The model under review builds one solid part; all positions refer to its coordinate system, in mm. Face numbers are marked on the shaded views. A direction names the side the tool comes from. Coordinates: 2 decimals unless noted, no trailing zeros. Order: outer loops, then holes, each group sorted by start corner. A loop starts at its lowest first (then second) coordinate and runs counter-clockwise, first axis right, second up. Notation, with made-up numbers: (86, 17) -> (130, 17) arc R11 cw to (130, 31) -> close; hole circle Ø11 at (32.5, 51). An arc over 180 degrees is marked (long way). Use CSV: the item, a comma, the result in double quotes. Start each with the question number.
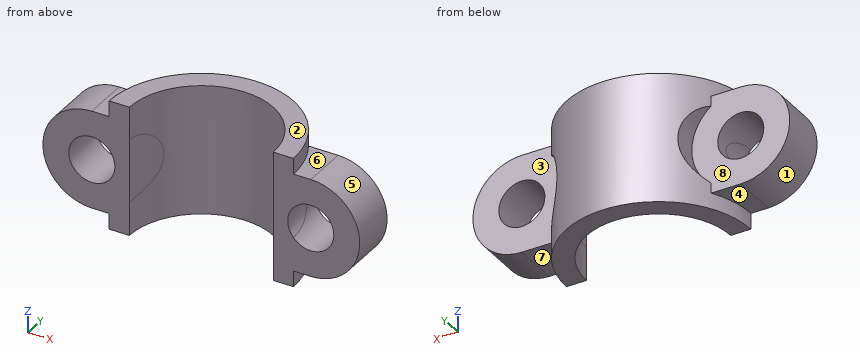
```python
from build123d import *

# Parameters (mm, degrees)
SKETCH_4_R          = 8.5
SKETCH_4_R_2        = 4
EXTRUDE_1_DEPTH     = 8
EXTRUDE_1_2_DEPTH   = 8
SKETCH_5_R          = 12.5
CUT_EXTRUDE_1_DEPTH = 10
EXTRUDE_3_DEPTH     = 11.25
SKETCH_7_R          = 8.5
CUT_EXTRUDE_2_DEPTH = 31.770318642
EXTRUDE_START       = -8
EXTRUDE_4_DEPTH     = 8
SKETCH_9_R          = 4
CUT_EXTRUDE_3_DEPTH = 31.770318642


with BuildPart() as part:
    # Sketch 4 → Extrude 1 (new body)
    with BuildSketch(Plane(origin=(0, 0, 0), x_dir=(1, 0, 0), z_dir=(0, 1, 0))):
        with Locations(Location((-19, 0, 0), (0, 0, 270))):
            Circle(SKETCH_4_R)
        with Locations(Location((-19, 0, 0), (0, 0, 270))):
            Circle(SKETCH_4_R_2, mode=Mode.SUBTRACT)
    extrude(amount=EXTRUDE_1_DEPTH)


with BuildPart() as body_2:
    # Sketch 4 → Extrude 1 2 (new body)
    with BuildSketch(Plane(origin=(0, 0, 0), x_dir=(1, 0, 0), z_dir=(0, 1, 0))):
        with Locations(Location((19, 0, 0), (0, 0, 90))):
            Circle(SKETCH_4_R)
        with Locations(Location((19, 0, 0), (0, 0, 90))):
            Circle(SKETCH_4_R_2, mode=Mode.SUBTRACT)
    extrude(amount=EXTRUDE_1_2_DEPTH)


with BuildPart() as cut_extrude_1_tool:
    # Sketch 5 → Cut-Extrude 1 (new, symmetric)
    with BuildSketch(Plane.XY):
        Circle(SKETCH_5_R)
    extrude(amount=CUT_EXTRUDE_1_DEPTH, both=True)


with BuildPart() as part_1:
    add(part.part)

    # Cut-Extrude 1: cut by cut_extrude_1_tool
    add(cut_extrude_1_tool.part, mode=Mode.SUBTRACT)



with BuildPart() as body_2_1:
    add(body_2.part)

    # Cut-Extrude 1: cut by cut_extrude_1_tool
    add(cut_extrude_1_tool.part, mode=Mode.SUBTRACT)


with BuildPart() as part_2:
    add(part_1.part)

    add(body_2_1.part)  # Extrude 3 merges body 2
    # Sketch 6 → Extrude 3 (add, symmetric)
    with BuildSketch(Plane.XY):
        with BuildLine():
            Line((-16, 0), (-12.5, 0))
            ThreePointArc((-12.5, 0), (0, 12.5), (12.5, 0))
            Line((12.5, 0), (16, 0))
            ThreePointArc((16, 0), (0, 16), (-16, 0))
        make_face()
    extrude(amount=EXTRUDE_3_DEPTH, both=True)

    # Sketch 7 → Cut-Extrude 2 (cut, through all)
    with BuildSketch(Plane(origin=(0, 8, 0), x_dir=(1, 0, 0), z_dir=(0, 1, 0))):
        with Locations((-19, 0)):
            Circle(SKETCH_7_R)
    cut_extrude_2 = extrude(amount=CUT_EXTRUDE_2_DEPTH, mode=Mode.SUBTRACT)

    # Sketch 8 → Extrude 4 (add)
    with BuildSketch(Plane(origin=(0, 8, 0), x_dir=(1, 0, 0), z_dir=(0, 1, 0)).offset(EXTRUDE_START)):
        with BuildLine():
            Line((-19, -8.5), (-19, -4))
            ThreePointArc((-19, -4), (-15, 0), (-19, 4))
            Line((-19, 4), (-19, 8.5))
            Line((-19, 8.5), (-13.461758669, 8.5))
            Line((-13.461758669, 8.5), (-13.461758669, -8.5))
            Line((-13.461758669, -8.5), (-19, -8.5))
        make_face()
    extrude_4 = extrude(amount=EXTRUDE_4_DEPTH)

    # Sketch 9 → Cut-Extrude 3 (cut, through all)
    with BuildSketch(Plane(origin=(0, 8, 0), x_dir=(1, 0, 0), z_dir=(0, 1, 0))):
        with Locations(Location((-19, 0, 0), (0, 0, 270))):
            Circle(SKETCH_9_R)
    cut_extrude_3 = extrude(amount=-CUT_EXTRUDE_3_DEPTH, mode=Mode.SUBTRACT)

    # Mirror 1: Cut-Extrude 2, Extrude 4, Cut-Extrude 3 across plane
    add(cut_extrude_2.mirror(Plane(origin=(0, 0, 0), x_dir=(0, 0, 1), z_dir=(1, 0, 0))), mode=Mode.SUBTRACT)
    add(extrude_4.mirror(Plane(origin=(0, 0, 0), x_dir=(0, 0, 1), z_dir=(1, 0, 0))))
    add(cut_extrude_3.mirror(Plane(origin=(0, 0, 0), x_dir=(0, 0, 1), z_dir=(1, 0, 0))), mode=Mode.SUBTRACT)


solid = part_2.part
```
Q1. Add section A-A, the plane z = 0. State the section outline as (x, y) points.
Q2. Add section C-C, the plane x = 0. State the section outline as (y, z) points, then the cut area to 4 significant figures.
Q3. Clearance check with flat-ended pins moving along their axes: pin 1 Ø2.5 at (x, y) = (16.5, 3.5) entering from +Z; pin 2 Ø5 at (x, z) = (20.5, 4) entering from +Y; pin 3 Ø1.5 at (x, y) = (-16.5, 5) entering from -Z; pin 4 Ø6 at (x, z) = (-5, 0) entering from +Y. State where each tip first meets the part, or that it passes through.
Q4. To check wall thickness, follow probe 1 along Z at (x, y) = (-19, 2.5); probe 2 along X at (y, z) = (2.75, 0.75); probe 3 along X at (y, z) = (5.25, 0). State the ranges of each line that lie inside material, in increasing order.
Q5. For the marked faces 4, 5, 6, 7 and 8, list the 3-axis set-ups (+Z, -Z, +X, -X, +Y, -Y) from which the entire face can be reached by the end or side of a thin tool; tool diameter is ignored.
Q6. Add section D-D, the plane y = 10.75. State the section outline as (x, z) points, then the cut area to 3 significant figures.
Q7. Draft analysis for pull direction Z (two halves, no side actions). For the marked faces 1, 2 and 3, state which applies: +Z half, -Z half, draft (parallel to the pull), parting line (faces both ways), or undercut.
Q8. Add section B-B, the plane y = 3. State the section outline as (x, z) points.
Answer block:
1,outline,"(-27.5, 0) -> (-23, 0) -> (-23, 8) -> (-27.5, 8) -> close; (-15, 0) -> (-12.5, 0) arc R12.5 cw to (12.5, 0) -> (15, 0) -> (15, 8) -> (10.5, 8) -> (10.5, 12.07) arc R16 ccw to (-10.5, 12.07) -> (-10.5, 8) -> (-15, 8) -> close; (23, 0) -> (27.5, 0) -> (27.5, 8) -> (23, 8) -> close"
2,outline,"(12.5, -11.25) -> (16, -11.25) -> (16, 11.25) -> (12.5, 11.25) -> close"
2,area,"78.75 mm²"
3,pin 1,"stops at z = 11.25"
3,pin 2,"stops at y = 8"
3,pin 3,"stops at z = -8.5"
3,pin 4,"stops at y = 15.87"
4,probe 1,"z = -8.5 to -4, 4 to 8.5"
4,probe 2,"x = -27.47 to -22.93, -15.07 to -12.19, 12.19 to 15.07, 22.93 to 27.47"
4,probe 3,"x = -27.5 to -23, -15 to -11.34, 11.34 to 15, 23 to 27.5"
5,face 4,"-Z, -X, +Y"
5,face 5,"+X, +Y, -Y"
5,face 6,"+Z, +X, +Y"
5,face 7,"-Z, +X, +Y"
5,face 8,"-X, +Y"
6,outline,"(-11.85, -11.25) -> (-6.38, -11.25) -> (-6.38, 11.25) -> (-11.85, 11.25) -> (-11.85, 4.6) arc R8.5 cw to (-11.85, -4.6) -> close; (6.38, -11.25) -> (11.85, -11.25) -> (11.85, -4.6) arc R8.5 cw to (11.85, 4.6) -> (11.85, 11.25) -> (6.38, 11.25) -> close"
6,area,"229 mm²"
7,face 1,"parting line"
7,face 2,"+Z half"
7,face 3,"undercut"
8,outline,"(-19, -8.5) -> (-15.72, -8.5) -> (-15.72, -11.25) -> (-12.13, -11.25) -> (-12.13, 11.25) -> (-15.72, 11.25) -> (-15.72, 8.5) -> (-19, 8.5) arc R8.5 ccw to start; (12.13, -11.25) -> (15.72, -11.25) -> (15.72, -8.5) -> (19, -8.5) arc R8.5 ccw to (19, 8.5) -> (15.72, 8.5) -> (15.72, 11.25) -> (12.13, 11.25) -> close; hole circle Ø8 at (-19, 0); hole circle Ø8 at (19, 0)"
